```python
from build123d import *

# Parameters (mm, degrees)
F1_DEPTH = 25


with BuildPart() as f1:
    # F0 (on Front) → F1 (new body)
    with BuildSketch(Plane.XZ):
        Polygon((3.464102, 10), (0.574671, 4.99536), (-3.464102, -2), (18.464102, -2), (14.425329, 4.99536), (11.535898, 10), (14.522771, 15.173416), (18.464102, 22), (-3.464102, 22), (-0.201125, 16.348359), align=None)
        Polygon((15, 0), (0, 0), (5.773503, 10), (0, 20), (15, 20), (9.226497, 10), align=None, mode=Mode.SUBTRACT)
    extrude(amount=F1_DEPTH)


solid = f1.part
```
For this review, take the finished solid that the model builds, in its own axes (mm). A direction names the side the tool comes from. Give positions to 0.01 mm unless a question says otherwise; leave off trailing zeros. Write each loop counter-clockwise with the first axis right and the second up, starting at its lowest first coordinate (ties: lowest second). Pieces come first, ordered by that corner, then holes. Notation, with made-up numbers: M 1,25 L 50,25 A14 cw 50,36 Z; hole C 84,18 d1. An arc over 180 degrees is marked long. One line per item, written item: value.
1) For faces 1 (the flat face through (7, -12, 20)), 2 (the flat face through (10, 0, 10)), list the 3-axis set-ups (+Z, -Z, +X, -X, +Y, -Y) from which the entire face can be reached by the end or side of a thin tool; tool diameter is ignored.
Results are:
face 1: +Y, -Y
face 2: +Z, -Z, +X, -X, +Y
2) Take a section at B-B, the plane x = 7.5. Write out the cut boundary in (y, z).
Results are:
outline: M -25,-2 L 0,-2 L 0,0 L -25,0 Z; M -25,20 L 0,20 L 0,22 L -25,22 Z
3) Take a section at D-D, the plane z = 4. Write out the cut boundary in (x, y), then the cut area to 3 significant figures.
Results are:
outline: M 0,-25 L 2.31,-25 L 2.31,0 L 0,0 Z; M 12.69,-25 L 15,-25 L 15,0 L 12.69,0 Z
area: 115 mm²
4) Take a section at A-A, the plane y = -11.5. Write out the cut boundary in (x, z), then the cut area to 3 significant figures.
Results are:
outline: M -3.46,-2 L 18.46,-2 L 14.43,5 L 11.54,10 L 14.52,15.17 L 18.46,22 L -3.46,22 L 3.46,10 L 0.57,5 Z; hole M 0,0 L 15,0 L 9.23,10 L 15,20 L 0,20 L 5.77,10 Z
area: 175 mm²
5) For P1, Ø6, axis at y = -12.5, z = 1.5, coming from the +X side; P2, Ø8, axis at y = -17, z = 1, coming from the -X side, all flat-tipped, find the tip position at first contact; note any pin that passes through.
Results are:
P1: stops at x = 18.18
P2: stops at x = -3.46
6) Take a section at C-C, the plane x = 10. Write out the cut boundary in (y, z).
Results are:
outline: M -25,-2 L 0,-2 L 0,0 L -25,0 Z; M -25,8.66 L 0,8.66 L 0,11.34 L -25,11.34 Z; M -25,20 L 0,20 L 0,22 L -25,22 Z
7) For line 1 (Z direction, x = 10.25, y = -9); line 2 (Z direction, x = 5.5, y = -19); line 3 (Z direction, x = 1, y = -16.5), list the stretches that pass through material, from the lowest coordinate up. Write a range as from..to.
Results are:
line 1: z = -2..0, 8.23..11.77, 20..22
line 2: z = -2..0, 9.53..10.47, 20..22
line 3: z = -2..0, 1.73..5.73, 14.27..18.27, 20..22
